CAD build for the part. Positions are in the model's coordinates, mm. Give positions to 0.01 mm unless a question says otherwise; leave off trailing zeros. Order: outer loops, then holes, each group sorted by start corner. A loop starts at its lowest first (then second) coordinate and runs counter-clockwise, first axis right, second up.
from build123d import *

# Parameters (mm, degrees)
BOSS_EXTRUDE1_DEPTH     = 32.766
SKETCH2_R               = 23.495
CUT_EXTRUDE1_DEPTH      = 52.487641673
M3_5X0_6_TAPPED_HOLE1_D = 2.9


with BuildPart() as part:
    # Sketch1 → Boss-Extrude1 (new body)
    with BuildSketch(Plane(origin=(0, 0, 0), x_dir=(0, 0, -1), z_dir=(1, 0, 0))):
        with BuildLine():
            Line((28.1, -18.939080971), (28.1, 18.939080971))
            ThreePointArc((28.1, 18.939080971), (27.799547486, 19.402749), (27.25359039, 19.317951577))
            ThreePointArc((27.25359039, 19.317951577), (19.564667335, 19.532372578), (19.341179036, 27.221037422))
            ThreePointArc((19.341179036, 27.221037422), (19.425455181, 27.766820849), (18.961909612, 28.067))
            Line((18.961909612, 28.067), (-18.961909612, 28.067))
            ThreePointArc((-18.961909612, 28.067), (-19.425455181, 27.766820849), (-19.341179036, 27.221037422))
            ThreePointArc((-19.341179036, 27.221037422), (-19.564667335, 19.532372578), (-27.25359039, 19.317951577))
            ThreePointArc((-27.25359039, 19.317951577), (-27.799547486, 19.402749), (-28.1, 18.939080971))
            Line((-28.1, 18.939080971), (-28.1, -18.939080971))
            ThreePointArc((-28.1, -18.939080971), (-27.799547486, -19.402749), (-27.25359039, -19.317951577))
            ThreePointArc((-27.25359039, -19.317951577), (-19.564667335, -19.532372578), (-19.341179036, -27.221037422))
            ThreePointArc((-19.341179036, -27.221037422), (-19.425455181, -27.766820849), (-18.961909612, -28.067))
            Line((-18.961909612, -28.067), (18.961909612, -28.067))
            ThreePointArc((18.961909612, -28.067), (19.425455181, -27.766820849), (19.341179036, -27.221037422))
            ThreePointArc((19.341179036, -27.221037422), (19.564667335, -19.532372578), (27.25359039, -19.317951577))
            ThreePointArc((27.25359039, -19.317951577), (27.799547486, -19.402749), (28.1, -18.939080971))
        make_face()
    extrude(amount=BOSS_EXTRUDE1_DEPTH)

    # Sketch2 → Cut-Extrude1 (cut, through all)
    with BuildSketch(Plane.ZY):
        Circle(SKETCH2_R)
    extrude(amount=-CUT_EXTRUDE1_DEPTH, mode=Mode.SUBTRACT)

    # M3.5x0.6 Tapped Hole1 (through all)
    with Locations(Plane(origin=(32.766, 0, 0), x_dir=(0, 0, -1), z_dir=(1, 0, 0))):
        with Locations((25.6794, 15.544299782), (25.6794, -15.544299782), (-25.6794, 15.544299782), (-25.6794, -15.544299782)):
            Hole(M3_5X0_6_TAPPED_HOLE1_D / 2)


solid = part.part
1. Saw through at C-C on x = 30.5. Give the cut face in (y, z) (3 decimals), plus the area to 3 significant figures.
2. Wall check: line 1 (Y direction, x = 3, z = -25.5); line 2 (Z direction, x = 29.5, y = 0.5); line 3 (Y direction, x = 12, z = 5). Give the ranges that are in metal, low to high.
3. Pin check, flat tips, straight feed: P1, Ø5, axis at y = -22, z = -3.5, coming from the -X side; P2, Ø2.5, axis at y = 15.54, z = -25.68, coming from the +X side. Stop position of each tip, or through.
4. Saw through at A-A on z = 0. Give the cut face in (x, y) (3 decimals), plus the area to 3 significant figures.
5. Mould opens along Y. For faces 1 (the flat face through (0, 17, -17)), 2 (the flat face through (16, -28.067, 0)), 3 (the cylindrical face through (16.2, 19.6, 19.5)) say: released by +Y, released by -Y, zero draft, split by the parting line, or undercut.
6. Saw through at B-B on y = 0. Give the cut face in (x, z) (3 decimals), plus the area to 3 significant figures.
Reported:
1. outline: (-28.067, -18.962) arc R0.508 ccw to (-27.221, -19.341) arc R5.601 cw to (-19.318, -27.254) arc R0.508 ccw to (-18.939, -28.1) - (18.939, -28.1) arc R0.508 ccw to (19.318, -27.254) arc R5.601 cw to (27.221, -19.341) arc R0.508 ccw to (28.067, -18.962) - (28.067, 18.962) arc R0.508 ccw to (27.221, 19.341) arc R5.601 cw to (19.318, 27.254) arc R0.508 ccw to (18.939, 28.1) - (-18.939, 28.1) arc R0.508 ccw to (-19.318, 27.254) arc R5.601 cw to (-27.221, 19.341) arc R0.508 ccw to (-28.067, 18.962) - close; hole circle Ø46.99 at (0, 0); hole circle Ø2.9 at (-15.544, -25.679); hole circle Ø2.9 at (-15.544, 25.679); hole circle Ø2.9 at (15.544, -25.679); hole circle Ø2.9 at (15.544, 25.679)
1. area: 1,030 mm2
2. line 1: y = -18.25 to -16.98, -14.11 to 14.11, 16.98 to 18.25
2. line 2: z = -28.1 to -23.49, 23.49 to 28.1
2. line 3: y = -28.07 to -22.96, 22.96 to 28.07
3. P1: stops at x = 0
3. P2: passes through
4. outline: (0, -28.067) - (32.766, -28.067) - (32.766, -23.495) - (0, -23.495) - close; (0, 23.495) - (32.766, 23.495) - (32.766, 28.067) - (0, 28.067) - close
4. area: 300 mm2
5. face 1: zero draft
5. face 2: released by -Y
5. face 3: undercut
6. outline: (0, -28.1) - (32.766, -28.1) - (32.766, -23.495) - (0, -23.495) - close; (0, 23.495) - (32.766, 23.495) - (32.766, 28.1) - (0, 28.1) - close
6. area: 302 mm2
